```python
from build123d import *


with BuildPart() as part:
    # Sketch1 → Revolve1 (revolve)
    with BuildSketch(Plane(origin=(0, 0, 0), x_dir=(0, 0, -1), z_dir=(1, 0, 0))):
        with BuildLine():
            Line((-2.5, 5.15), (-2.5, 4))
            Line((-2.5, 4), (2.5, 4))
            Line((2.5, 4), (2.5, 5.15))
            Line((2.5, 5.15), (2.25, 5.15))
            Line((2.25, 5.15), (2.25, 5.3))
            Line((2.25, 5.3), (0.714142843, 5.3))
            ThreePointArc((0.714142843, 5.3), (0, 5), (-0.714142843, 5.3))
            Line((-0.714142843, 5.3), (-2.25, 5.3))
            Line((-2.25, 5.3), (-2.25, 5.15))
            Line((-2.25, 5.15), (-2.5, 5.15))
        make_face()
    revolve(axis=Axis((0, 0, 6.755399071), (0, 0, -1)))


solid = part.part
```
The listing builds one solid part. Answer for the finished solid, in the listing's coordinates (mm). Coordinates: 2 decimals unless noted, no trailing zeros. Loops run counter-clockwise (first coordinate to the right, second up) from the corner with the lowest first, then second, coordinate; pieces in that order, holes last. Notation, with made-up numbers: M 42.5,89.5 L 92.5,89.5 A6 cw 92.5,95.5 Z; hole C -23,-9.5 d9. An arc over 180 degrees is marked long. Answer as a JSON object with one key per item and string values. Group by question number.
Item 1: Section A-A (y = 0) is taken. Write down the section's boundary in (x, z), and give its area (3 significant figures).
Item 2: Each of these flat-tipped pins is pushed along its axis until it touches: P1, Ø1, axis at y = 2, z = 0.5, coming from the +X side; P2, Ø1.5, axis at y = -4, z = 1, coming from the -X side; P3, Ø3, axis at y = 2, z = -0.5, coming from the -X side. Where does it stop, or does it pass through?
Item 3: Determine the mould class of faces 1 (the face through (-3.905, -0.867, -0.035)), 2 (the face through (-2.03, 4.896, 1.493)), 3 (the face through (-3, -3, -2.5)) for opening direction Y: +Y half, -Y half, draft (parallel to the pull), parting line (faces both ways), or undercut.
Item 4: Consider L1, parallel to X at y = 0, z = 1.2; L2, parallel to X at y = 0, z = 0.2; L3, parallel to Y at x = -0.75, z = -0.75. Determine where each line is inside the solid, lowest interval first.
Item 5: Section D-D (z = 0.1) is taken. Write down the section's boundary in (x, y), and give its area (3 significant figures).
Item 6: Section C-C (z = -1) is taken. Write down the section's boundary in (x, y), and give its area (3 significant figures).
Solved:
{
 "1": {"outline": "M -5.3,-2.25 L -5.15,-2.25 L -5.15,-2.5 L -4,-2.5 L -4,2.5 L -5.15,2.5 L -5.15,2.25 L -5.3,2.25 L -5.3,0.71 A1 cw -5.3,-0.71 Z; M 4,-2.5 L 5.15,-2.5 L 5.15,-2.25 L 5.3,-2.25 L 5.3,-0.71 A1 cw 5.3,0.71 L 5.3,2.25 L 5.15,2.25 L 5.15,2.5 L 4,2.5 Z", "area": "12.3 mm2"},
 "2": {"P1": "stops at x = 5.07", "P2": "stops at x = -4.19", "P3": "stops at x = -5.27"},
 "3": {"face 1": "undercut", "face 2": "parting line", "face 3": "draft"},
 "4": {"L1": "x = -5.3 to -4, 4 to 5.3", "L2": "x = -5.02 to -4, 4 to 5.02", "L3": "y = -5.25 to -3.93, 3.93 to 5.25"},
 "5": {"outline": "C 0,0 d10.01; hole C 0,0 d8", "area": "28.4 mm2"},
 "6": {"outline": "C 0,0 d10.6; hole C 0,0 d8", "area": "38.0 mm2"}
}
